```python
from build123d import *

# Parameters (mm, degrees)
SKETCH2_R           = 1.75
BOSS_EXTRUDE1_DEPTH = 30
BOSS_EXTRUDE2_DEPTH = 32
SKETCH6_R           = 3
CUT_EXTRUDE3_DEPTH  = 28
SKETCH7_W           = 0.45
SKETCH7_H           = 28
CUT_EXTRUDE4_DEPTH  = 13
SKETCH8_R           = 1.25
CUT_EXTRUDE5_DEPTH  = 5.39427731
SKETCH8_3_R         = 1.25
CUT_EXTRUDE6_DEPTH  = 6.291522586


with BuildPart() as part:
    # Sketch2 → Boss-Extrude1 (new body)
    with BuildSketch(Plane(origin=(0, 0, 0), x_dir=(1, 0, 0), z_dir=(0, 1, 0))):
        with BuildLine():
            Line((-24.821747911, -3.435069212), (-12.987160246, -2.166440487))
            ThreePointArc((-12.987160246, -2.166440487), (-10.8566751, -0.059524017), (-12.939762178, 2.094266176))
            Line((-12.939762178, 2.094266176), (-24.821781773, 3.29179515))
            ThreePointArc((-24.821781773, 3.29179515), (-30.987291256, -0.071668068), (-24.821747911, -3.435069212))
        make_face()
        with Locations((-26.987114413, 0)):
            Circle(SKETCH2_R, mode=Mode.SUBTRACT)
    extrude(amount=BOSS_EXTRUDE1_DEPTH)

    # Sketch2_3 → Boss-Extrude2 (add)
    with BuildSketch(Plane(origin=(0, 0, 0), x_dir=(1, 0, 0), z_dir=(0, 1, 0))):
        with BuildLine():
            ThreePointArc((-26.987114411, 4.428185187), (-31.48694753, -0.071647931), (-26.987114411, -4.57148105))
            Line((-26.987114411, -4.57148105), (-12.987160246, -2.67247066))
            ThreePointArc((-12.987160246, -2.67247066), (-11.181747177, -1.957383249), (-10.355629468, -0.2))
            Line((-10.355629468, -0.2), (-10.371987074, 0.3))
            ThreePointArc((-10.371987074, 0.3), (-11.245543176, 1.943741621), (-12.987160246, 2.600823626))
            Line((-12.987160246, 2.600823626), (-26.987114411, 4.428185187))
        make_face()
        with BuildLine():
            ThreePointArc((-24.821747911, -3.435069212), (-30.987291256, -0.071668068), (-24.821781773, 3.29179515))
            Line((-24.821781773, 3.29179515), (-12.939762178, 2.094266176))
            ThreePointArc((-12.939762178, 2.094266176), (-10.8566751, -0.059524017), (-12.987160246, -2.166440487))
            Line((-12.987160246, -2.166440487), (-24.821747911, -3.435069212))
        make_face(mode=Mode.SUBTRACT)
    extrude(amount=BOSS_EXTRUDE2_DEPTH)

    # Sketch6 → Cut-Extrude3 (cut)
    with BuildSketch(Plane.XZ):
        with Locations((-26.987114413, 0)):
            Circle(SKETCH6_R)
    extrude(amount=-CUT_EXTRUDE3_DEPTH, mode=Mode.SUBTRACT)

    # Sketch7 → Cut-Extrude4 (cut)
    with BuildSketch(Plane(origin=(-10.351093889, 0, 0.338638235), x_dir=(-0.032697719, 0, -0.999465287), z_dir=(0.999465287, 0, -0.032697719))):
        with Locations((0.388846156, 15)):
            Rectangle(SKETCH7_W, SKETCH7_H)
    extrude(amount=-CUT_EXTRUDE4_DEPTH, mode=Mode.SUBTRACT)

    # Sketch8 → Cut-Extrude5 (cut, through all)
    with BuildSketch(Plane(origin=(-0.005357396, 0, -0.163758545), x_dir=(-0.999465287, 0, 0.032697719), z_dir=(-0.032697719, 0, -0.999465287))):
        with Locations((12.895174838, 28.5)):
            Circle(SKETCH8_R)
        with Locations((12.895174838, 1.5)):
            Circle(SKETCH8_R)
    extrude(amount=-CUT_EXTRUDE5_DEPTH, mode=Mode.SUBTRACT)

    # Sketch8_3 → Cut-Extrude6 (cut, through all)
    with BuildSketch(Plane(origin=(-0.005357396, 0, -0.163758545), x_dir=(-0.999465287, 0, 0.032697719), z_dir=(-0.032697719, 0, -0.999465287))):
        with Locations((12.895174838, 28.5)):
            Circle(SKETCH8_3_R)
        with Locations((12.895174838, 1.5)):
            Circle(SKETCH8_3_R)
    extrude(amount=CUT_EXTRUDE6_DEPTH, mode=Mode.SUBTRACT)


solid = part.part
```
Build history of the part. All positions in model axes, mm. A direction names the side the tool comes from. Round coordinates to 2 decimals unless told otherwise and drop trailing zeros.
Item 1: Two-plate mould, pull along Z, no slides. Class faces 4 (the face through (-27, 28, -2)), 5 (the face through (-19.89, 15.78, -3.5)), 6 (the face through (-31.486, 15.776, -0.027)): released by +Z, released by -Z, zero draft, split by the parting line, or undercut.
Item 2: Drill centre lines: line 1 along Y through (x, z) = (-13.5, -0.25); line 2 along X through (y, z) = (29.45, 0); line 3 along Y through (x, z) = (-22, 0). Where is each one in solid material? Low to high.
Item 3: Pin check, flat tips, straight feed: P1, Ø0.8, axis at x = -18.5, z = 0, coming from the +Y side; P2, Ø3, axis at x = -17.5, y = 3.5, coming from the +Z side; P3, Ø1.8, axis at x = -28, z = 0.5, coming from the -Y side. Stop position of each tip, or through.
Item 4: Which spindle directions (+Z, -Z, +X, -X, +Y, -Y) get a long thin tool onto all of the face, cutting with end or side? Do faces 1 (the face through (-24.216, 13.804, -1.149)), 2 (the face through (-18.82, 30.99, 2.79)), 3 (the face through (-20.085, 15.776, 3.635)). Say none if no direction does.
Worked answers:
1. face 4: undercut
1. face 5: released by -Z
1. face 6: split by the parting line
2. line 1: y = 0 to 0.4, 2.6 to 27.4, 29.6 to 30
2. line 2: x = -31.49 to -28.74, -25.24 to -13.71, -12.09 to -10.36
2. line 3: y = 0 to 30
3. P1: stops at y = 30
3. P2: stops at z = 3.49
3. P3: stops at y = 28
4. face 1: -Y
4. face 2: +Y
4. face 3: +Z, +X, +Y, -Y
